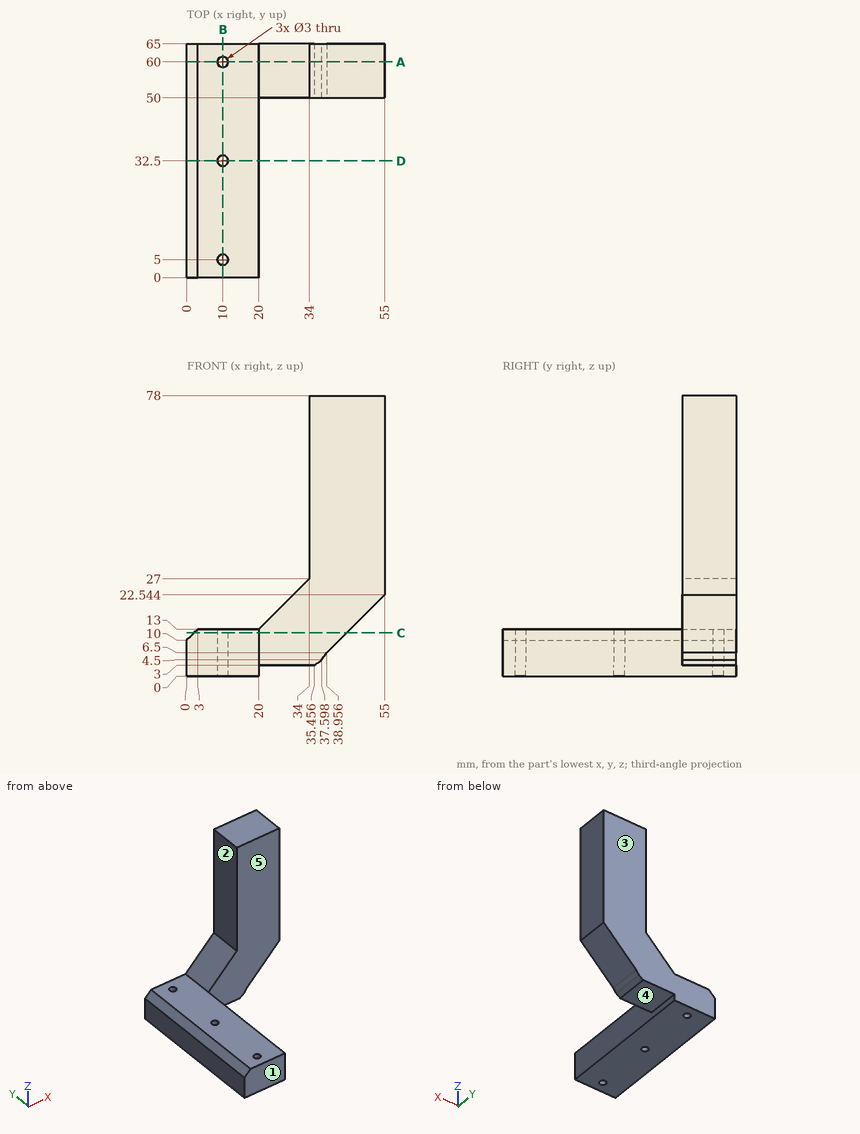
Design review of the part shown in the three views and the two pictorial views. Dimensions are in mm from the part's minimum x, y and z. A direction names the side the tool comes from. Round coordinates to 2 decimals unless told otherwise and drop trailing zeros. Loops run counter-clockwise (first coordinate to the right, second up) from the corner with the lowest first, then second, coordinate; pieces in that order, holes last.
(1) Clearance check with flat-ended pins moving along their axes: P1, Ø3, axis at y = 58, z = 69, coming from the -X side; P2, Ø5, axis at x = 10, y = 36.5, coming from the +Z side; P3, Ø6, axis at x = 45, z = 35.5, coming from the -Y side; P4, Ø2.5, axis at x = 10, y = 32.5, coming from the +Z side. State where each tip first meets the part, or that it passes through.
Returned:
P1: stops at x = 34
P2: stops at z = 13
P3: stops at y = 50
P4: passes through
(2) Wall thickness on line 1 along Y through (x, z) = (10, 1.6); line 2 along X through (y, z) = (60, 2.4); line 3 along Y through (x, z) = (47.5, 32): over which ranges is each line inside the solid? List them lowest first.
Returned:
line 1: y = 0 to 3.5, 6.5 to 31, 34 to 58.5, 61.5 to 65
line 2: x = 0 to 8.5, 11.5 to 20
line 3: y = 50 to 65
(3) We need section B-B (x = 10). Give the boundary of the cut face in (y, z), plus the area to 3 significant figures.
Returned:
outline: (0, 0) - (3.5, 0) - (3.5, 13) - (0, 13) - close; (6.5, 0) - (31, 0) - (31, 13) - (6.5, 13) - close; (34, 0) - (58.5, 0) - (58.5, 13) - (34, 13) - close; (61.5, 0) - (65, 0) - (65, 13) - (61.5, 13) - close
area: 728 mm2
(4) We need section A-A (y = 60). Give the boundary of the cut face in (x, z), plus the area to 3 significant figures.
Returned:
outline: (0, 0) - (8.5, 0) - (8.5, 13) - (3, 13) - (0, 10) - close; (11.5, 0) - (20, 0) - (20, 3) - (35.46, 3) - (37.6, 4.5) - (38.96, 6.5) - (55, 22.54) - (55, 78) - (34, 78) - (34, 27) - (20, 13) - (11.5, 13) - close
area: 1,840 mm2
(5) Mouldability with a two-part tool opening along Y and no side actions: class the marked faces 3, 4 and 5 as released by +Y, released by -Y, zero draft, split by the parting line, or undercut.
Returned:
face 3: released by +Y
face 4: zero draft
face 5: released by -Y
(6) Tool access review of the marked faces 1 and 2: name each direction out of +Z, -Z, +X, -X, +Y, -Y from which nothing blocks a thin tool from reaching the whole face with its end or side.
Returned:
face 1: +Z, -Z, +X, -X, -Y
face 2: +Z, -X, +Y, -Y
(7) We need section D-D (y = 32.5). Give the boundary of the cut face in (x, z), plus the area to 4 significant figures.
Returned:
outline: (0, 0) - (8.5, 0) - (8.5, 13) - (3, 13) - (0, 10) - close; (11.5, 0) - (20, 0) - (20, 13) - (11.5, 13) - close
area: 216.5 mm2
(8) We need section C-C (z = 12). Give the boundary of the cut face in (x, y).
Returned:
outline: (2, 0) - (20, 0) - (20, 50) - (44.46, 50) - (44.46, 65) - (2, 65) - close; hole circle Ø3 at (10, 5); hole circle Ø3 at (10, 32.5); hole circle Ø3 at (10, 60)
